```python
from build123d import *

# Parameters (mm, degrees)
SKETCH1_W             = 4.5
SKETCH1_H             = 4.5
BOSS_EXTRUDE1_DEPTH   = 50
BOSS_EXTRUDE1_2_DEPTH = 50
SKETCH2_W             = 4.5
SKETCH2_H             = 6
BOSS_EXTRUDE2_DEPTH   = 25
FILLET1_R             = 10
FILLET2_R             = 5
SKETCH5_W             = 4.5
SKETCH5_H             = 4
CUT_EXTRUDE3_DEPTH    = 2.75
SKETCH6_W             = 4.5
SKETCH6_H             = 4
CUT_EXTRUDE4_DEPTH    = 2.75
SKETCH3_W             = 4.5
SKETCH3_H             = 4
CUT_EXTRUDE1_DEPTH    = 2.5
SKETCH4_W             = 4.5
SKETCH4_H             = 4
CUT_EXTRUDE2_DEPTH    = 2.5


with BuildPart() as part:
    # Sketch1 → Boss-Extrude1 (new body)
    with BuildSketch(Plane(origin=(0, 0, 0), x_dir=(1, 0, 0), z_dir=(0, 1, 0))):
        with Locations((-18.391025641, 0.25)):
            Rectangle(SKETCH1_W, SKETCH1_H)
    extrude(amount=BOSS_EXTRUDE1_DEPTH)



with BuildPart() as body_2:
    # Sketch1 → Boss-Extrude1 2 (new body)
    with BuildSketch(Plane(origin=(0, 0, 0), x_dir=(1, 0, 0), z_dir=(0, 1, 0))):
        with Locations((10.458974359, 0.25)):
            Rectangle(SKETCH1_W, SKETCH1_H)
    extrude(amount=BOSS_EXTRUDE1_2_DEPTH)


with BuildPart() as part_1:
    add(part.part)

    add(body_2.part)  # Boss-Extrude2 merges body 2
    # Sketch2 → Boss-Extrude2 (add)
    with BuildSketch(Plane.ZY.offset(-8.208974359)):
        with Locations((-0.25, 47)):
            Rectangle(SKETCH2_W, SKETCH2_H)
    extrude(amount=BOSS_EXTRUDE2_DEPTH)

    # Fillet1
    fillet1_edges = [part_1.edges().sort_by_distance(p)[0] for p in [
        (-20.641025641, 50, -0.25),
        (12.708974359, 50, -0.25),
    ]]
    fillet(fillet1_edges, radius=FILLET1_R)

    # Fillet2
    fillet2_edges = [part_1.edges().sort_by_distance(p)[0] for p in [
        (-16.141025641, 44, -0.25),
        (8.208974359, 44, -0.25),
    ]]
    fillet(fillet2_edges, radius=FILLET2_R)

    # Sketch5 → Cut-Extrude3 (cut)
    with BuildSketch(Plane.XY.offset(2)):
        with Locations((10.458974359, 6)):
            Rectangle(SKETCH5_W, SKETCH5_H)
    extrude(amount=-CUT_EXTRUDE3_DEPTH, mode=Mode.SUBTRACT)

    # Sketch6 → Cut-Extrude4 (cut)
    with BuildSketch(Plane(origin=(0, 0, -2.5), x_dir=(-1, 0, 0), z_dir=(0, 0, -1))):
        with Locations((18.391025641, 6)):
            Rectangle(SKETCH6_W, SKETCH6_H)
    extrude(amount=-CUT_EXTRUDE4_DEPTH, mode=Mode.SUBTRACT)

    # Sketch3 → Cut-Extrude1 (cut)
    with BuildSketch(Plane.ZY.offset(-8.208974359)):
        with Locations((-0.25, 6)):
            Rectangle(SKETCH3_W, SKETCH3_H)
    extrude(amount=-CUT_EXTRUDE1_DEPTH, mode=Mode.SUBTRACT)

    # Sketch4 → Cut-Extrude2 (cut)
    with BuildSketch(Plane(origin=(-16.141025641, 0, 0), x_dir=(0, 0, -1), z_dir=(1, 0, 0))):
        with Locations((0.25, 6)):
            Rectangle(SKETCH4_W, SKETCH4_H)
    extrude(amount=-CUT_EXTRUDE2_DEPTH, mode=Mode.SUBTRACT)


solid = part_1.part
```
CAD build for the part. Positions are in the model's coordinates, mm. A direction names the side the tool comes from. Round coordinates to 2 decimals unless told otherwise and drop trailing zeros. Order: outer loops, then holes, each group sorted by start corner. A loop starts at its lowest first (then second) coordinate and runs counter-clockwise, first axis right, second up.
Q1. Slice it at A-A (z = -1.5). Write the cut outline in (x, y).
Q2. Two-plate mould, pull along Y, no slides. Class faces 4 (the flat face through (-18, 0, 0)), 5 (the flat face through (-20, 6, 0.25)), 6 (the flat face through (-16.141, 2, 0)): pulls with the +Y half, pulls with the -Y half, needs draft (parallel to the pull), parting line crosses it, or undercut.
Q3. Slice it at B-B (y = 7). Write the cut outline in (x, z).
Q4. Slice it at C-C (y = 34). Write the cut outline in (x, z).
Q5. Which spindle directions (+Z, -Z, +X, -X, +Y, -Y) get a long thin tool onto all of the face, cutting with end or side? Do faces 1 (the flat face through (-4, 44, 0)), 2 (the flat face through (10, 4, 0)), 3 (the flat face through (12, 6, -0.75)). Say none if no direction does.
Q6. Slice it at D-D (x = -5.5). Write the cut outline in (y, z), and give its area (3 significant figures).
Q7. Drop flat-ended pins along their axis: pin 1 (1.6 mm diameter, centred on x = 12, y = 6, fed in from +Z); pin 2 (2 mm diameter, centred on x = -2, z = 1, fed in from -Y); pin 3 (0.5 mm diameter, centred on y = 7, z = 1, fed in from +X). Give the stop position or say it passes through.
Q8. Wall check: L1, parallel to X at y = 21.5, z = 0.15; L2, parallel to Y at x = -3.5, z = -1.75; L3, parallel to Y at x = -18, z = -0.5. Give the ranges that are in metal, low to high.
Results below:
1. outline: (-20.64, 0) - (-16.14, 0) - (-16.14, 4) - (-20.64, 4) - close; (-20.64, 8) - (-16.14, 8) - (-16.14, 39) arc R5 cw to (-11.14, 44) - (3.21, 44) arc R5 cw to (8.21, 39) - (8.21, 8) - (10.71, 8) - (10.71, 4) - (8.21, 4) - (8.21, 0) - (12.71, 0) - (12.71, 40) arc R10 ccw to (2.71, 50) - (-10.64, 50) arc R10 ccw to (-20.64, 40) - close
2. face 4: pulls with the -Y half
2. face 5: undercut
2. face 6: needs draft
3. outline: (-20.64, 0.25) - (-18.64, 0.25) - (-18.64, 2) - (-20.64, 2) - close; (10.71, -2.5) - (12.71, -2.5) - (12.71, -0.75) - (10.71, -0.75) - close
4. outline: (-20.64, -2.5) - (-16.14, -2.5) - (-16.14, 2) - (-20.64, 2) - close; (8.21, -2.5) - (12.71, -2.5) - (12.71, 2) - (8.21, 2) - close
5. face 1: +Z, -Z, -Y
5. face 2: +Z
5. face 3: +Z, +X, -X
6. outline: (44, -2.5) - (50, -2.5) - (50, 2) - (44, 2) - close
6. area: 27.0 mm2
7. pin 1: stops at z = -0.75
7. pin 2: stops at y = 44
7. pin 3: stops at x = -18.64
8. L1: x = -20.64 to -16.14, 8.21 to 12.71
8. L2: y = 44 to 50
8. L3: y = 0 to 4, 8 to 46.77
